Design review of the part built by this model. Coordinates are the model's own, in mm. Round coordinates to 2 decimals unless told otherwise and drop trailing zeros. Order: outer loops, then holes, each group sorted by start corner. A loop starts at its lowest first (then second) coordinate and runs counter-clockwise, first axis right, second up. Notation, with made-up numbers: M 88.5,87.25 L 107.5,87.25 A13 ccw 107.5,103.25 Z; hole C 31,-15 d2. An arc over 180 degrees is marked long. Use a Markdown table: item, result. Add a question column.
(1) To check wall thickness, follow probe 1 along Y at (x, z) = (-47.5, 1.4); probe 2 along X at (y, z) = (7, 0.85); probe 3 along X at (y, z) = (59, 1.8). State the ranges of each line that lie inside material, in increasing order. Write a range as from..to.
(2) Take a section at C-C (z = 1.05). Write out the cut boundary in (x, y), then the cut area to 3 significant figures.
(3) For pin 1 (1 mm diameter, centred on x = 5.5, z = 0.5, fed in from -Y); pin 2 (0.6 mm diameter, centred on x = -26.5, z = 1.5, fed in from +Y); pin 3 (0.6 mm diameter, centred on x = -47, z = 0.5, fed in from -Y), all flat-tipped, find the tip position at first contact; note any pin that passes through.
(4) Take a section at A-A (x = -48). Write out the cut boundary in (y, z), then the cut area to 3 significant figures.
(5) Take a section at B-B (y = 35.5). Write out the cut boundary in (x, z).
(6) Take a section at D-D (y = -12.5). Write out the cut boundary in (x, z).
```python
from build123d import *

# Parameters (mm, degrees)
SKETCH_R  = 5
PAD_DEPTH = 2


with BuildPart() as part:
    # Sketch → Pad (new body)
    with BuildSketch(Plane.XY):
        with BuildLine():
            Line((-52.333898, 55.022503), (5.545685, 55.022503))
            ThreePointArc((21.389974, 36.795733), (17.621038, 49.519447), (5.545685, 55.022503))
            Line((13.074881, -22.369229), (21.389974, 36.795733))
            ThreePointArc((-6.14321, -24.613861), (4.332293, -30.909979), (13.074881, -22.369229))
            ThreePointArc((-6.14321, -24.613861), (-10.552788, -19.068824), (-17.321701, -16.977497))
            Line((-17.321701, -16.977497), (-66.8278, -16.977497))
            ThreePointArc((-82.8278, -0.977497), (-78.141508, -12.291206), (-66.8278, -16.977497))
            Line((-82.8278, -0.977497), (-82.8278, 59.022503))
            ThreePointArc((-63.51239, 62.658866), (-74.677922, 68.849865), (-82.8278, 59.022503))
            ThreePointArc((-63.51239, 62.658866), (-59.102811, 57.113829), (-52.333898, 55.022503))
        make_face()
        with Locations((3.1722, -20.977497)):
            Circle(SKETCH_R, mode=Mode.SUBTRACT)
        with Locations((-72.8278, 59.022503)):
            Circle(SKETCH_R, mode=Mode.SUBTRACT)
        with BuildLine():
            Line((-64.8278, 49.022503), (5.545685, 49.022503))
            ThreePointArc((15.448366, 37.630771), (13.092781, 45.583093), (5.545685, 49.022503))
            Line((15.448366, 37.630771), (11.520471, 9.682348))
            ThreePointArc((-12.245963, -10.977497), (3.499454, -5.090527), (11.520471, 9.682348))
            Line((-12.245963, -10.977497), (-66.8278, -10.977497))
            ThreePointArc((-76.8278, -0.977497), (-73.898868, -8.048565), (-66.8278, -10.977497))
            Line((-76.8278, -0.977497), (-76.8278, 37.022503))
            ThreePointArc((-64.8278, 49.022503), (-73.313081, 45.507784), (-76.8278, 37.022503))
        make_face(mode=Mode.SUBTRACT)
    extrude(amount=PAD_DEPTH)


solid = part.part
```
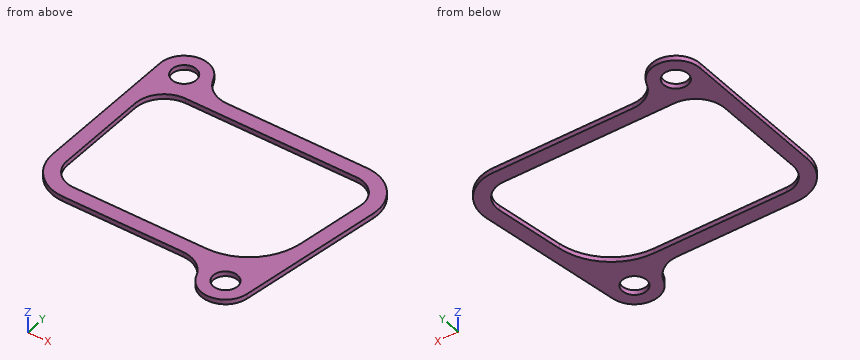
Verdict:
| question | item | result |
|---|---|---|
| 1 | probe 1 | y = -16.98..-10.98, 49.02..55.02 |
| 1 | probe 2 | x = -82.83..-76.83, 10.99..17.2 |
| 1 | probe 3 | x = -82.83..-77.83, -67.83..-61.26 |
| 2 | outline | M -82.83,-0.98 A16 ccw -66.83,-16.98 L -17.32,-16.98 A12 cw -6.14,-24.61 A10 ccw 13.07,-22.37 L 21.39,36.8 A16 ccw 5.55,55.02 L -52.33,55.02 A12 cw -63.51,62.66 A10 ccw -82.83,59.02 Z; hole C -72.83,59.02 d10; hole M -76.83,-0.98 A10 ccw -66.83,-10.98 L -12.25,-10.98 A24 ccw 11.52,9.68 L 15.45,37.63 A10 ccw 5.55,49.02 L -64.83,49.02 A12 ccw -76.83,37.02 Z; hole C 3.17,-20.98 d10 |
| 2 | area | 2,340 mm^2 |
| 3 | pin 1 | stops at y = -30.81 |
| 3 | pin 2 | stops at y = 55.02 |
| 3 | pin 3 | stops at y = -16.98 |
| 4 | outline | M -16.98,0 L -10.98,0 L -10.98,2 L -16.98,2 Z; M 49.02,0 L 55.02,0 L 55.02,2 L 49.02,2 Z |
| 4 | area | 24.0 mm^2 |
| 5 | outline | M -82.83,0 L -76.83,0 L -76.83,2 L -82.83,2 Z; M 15.15,0 L 21.21,0 L 21.21,2 L 15.15,2 Z |
| 6 | outline | M -77.93,0 L 14.46,0 L 14.46,2 L -77.93,2 Z |
